Here's how the part is built. I have some questions about the finished solid (model axes, mm). Face numbers are marked on the shaded views. Give positions to 0.01 mm unless a question says otherwise; leave off trailing zeros. Order: outer loops, then holes, each group sorted by start corner. A loop starts at its lowest first (then second) coordinate and runs counter-clockwise, first axis right, second up. Notation, with made-up numbers: (-9.75, 89.5) -> (35.25, 89.5) arc R18 ccw to (35.25, 121.5) -> close; hole circle Ø8 at (-23, 51). An arc over 180 degrees is marked (long way). Write each question's results on one line, items separated by ' | '. Start each with the question number.
Q1. I'm going to push flat-ended pins straight in: pin 1 (1.4 mm diameter, centred on x = 10.2, y = 5.063, fed in from +Z); pin 2 (3.5 mm diameter, centred on x = 6, y = 9.5, fed in from +Z). Where does each tip first touch, or does it pass through?
Q2. Imagine slicing it at B-B, the plane y = 29.21. Please give me the cut outline in (x, z).
Q3. I need wall thicknesses on line 1 along Y through (x, z) = (17.5, -1.1); line 2 along X through (y, z) = (1, -1.25); line 3 along Y through (x, z) = (2, -3.05). Which ranges of each line are inside material? Lowest first, please. Write a range as [from, to].
Q4. Imagine slicing it at D-D, the plane y = 13. Please give me the cut outline in (x, z), then the cut area to 3 significant figures.
Q5. Imagine slicing it at C-C, the plane z = -3.2. Please give me the cut outline in (x, y).
Q6. Imagine slicing it at A-A, the plane x = 22.86. Please give me the cut outline in (y, z).
Q7. Thinking about a two-plate mould opening in Z: for the marked faces 1, 2 and 3, which applies, pulls with the +Z half, pulls with the -Z half, needs draft (parallel to the pull), parting line crosses it, or undercut?
```python
from build123d import *

# Parameters (mm, degrees)
PAD_DEPTH       = 3.2
THICKNESS001_T  = -2
SKETCH010_R     = 1.25
POCKET002_DEPTH = 2.001
SKETCH011_R     = 1.5
SKETCH011_R_2   = 1.2
POCKET003_DEPTH = 1


with BuildPart() as part:
    # Sketch009 → Pad (new body)
    with BuildSketch(Plane.XY):
        with BuildLine():
            Line((-2.4, 31.749999), (-2.4, 0))
            ThreePointArc((-2.4, 0), (-1.697056, -1.697056), (0, -2.4))
            Line((0, -2.4), (25.4, -2.4))
            ThreePointArc((25.4, -2.4), (27.097056, -1.697057), (27.8, -1e-06))
            Line((27.8, -1e-06), (27.8, 31.75))
            ThreePointArc((27.8, 31.75), (27.097057, 33.447056), (25.400001, 34.15))
            Line((25.400001, 34.15), (1e-06, 34.15))
            ThreePointArc((1e-06, 34.15), (-1.697056, 33.447056), (-2.4, 31.749999))
        make_face()
    extrude(amount=PAD_DEPTH)

    # Thickness001
    thickness001_openings = [part.faces().sort_by_distance(p)[0] for p in [
        (12.7, 15.875, 3.2),
    ]]
    offset(amount=THICKNESS001_T, openings=thickness001_openings)

    # Sketch010 (on Face19 of Thickness001) → Pocket002 (cut, through all)
    with BuildSketch(Plane.XY.offset(2)):
        with Locations((2.54, 29.21)):
            Circle(SKETCH010_R)
        with Locations((22.86, 29.21)):
            Circle(SKETCH010_R)
        with Locations((22.86, 2.54)):
            Circle(SKETCH010_R)
        with Locations((2.54, 2.54)):
            Circle(SKETCH010_R)
    extrude(amount=-POCKET002_DEPTH, mode=Mode.SUBTRACT)

    # Sketch011 (on Face23 of Pocket002) → Pocket003 (cut)
    with BuildSketch(Plane.XY.offset(2)):
        with Locations((9.45, 24.043)):
            Circle(SKETCH011_R)
        with Locations((15.95, 24.043)):
            Circle(SKETCH011_R)
        with Locations((15.95, 19.543)):
            Circle(SKETCH011_R)
        with Locations((19.025, 18.793)):
            Circle(SKETCH011_R)
        with Locations((19.025, 8.793)):
            Circle(SKETCH011_R)
        with Locations((9.45, 19.543)):
            Circle(SKETCH011_R)
        with Locations((6.375, 18.793)):
            Circle(SKETCH011_R)
        with Locations((6.375, 8.793)):
            Circle(SKETCH011_R)
        with Locations((3.97, 16.293)):
            Circle(SKETCH011_R_2)
        with Locations((3.97, 13.793)):
            Circle(SKETCH011_R_2)
        with Locations((3.97, 11.293)):
            Circle(SKETCH011_R_2)
        with Locations((10.2, 5.063)):
            Circle(SKETCH011_R_2)
        with Locations((12.7, 5.063)):
            Circle(SKETCH011_R_2)
        with Locations((15.2, 5.063)):
            Circle(SKETCH011_R_2)
    extrude(amount=-POCKET003_DEPTH, mode=Mode.SUBTRACT)


with BuildPart() as part_1:
    # Body placement: moved
    add(part.part.moved(Location((0, 0, -3.6))))


solid = part_1.part
```
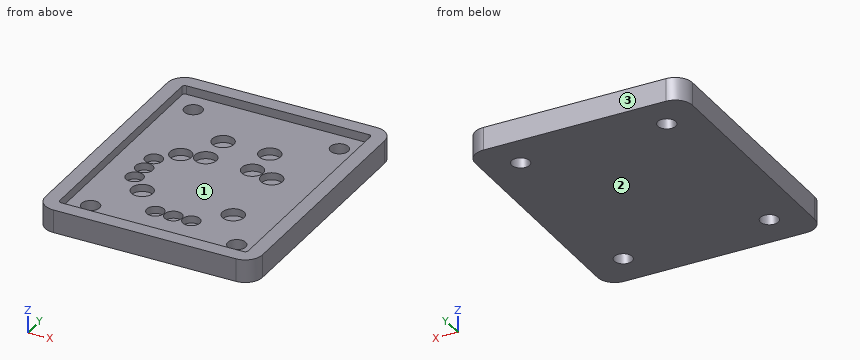
Geometry check:
1) pin 1: z = -2.6 | pin 2: z = -1.6
2) outline: (-2.4, -3.6) -> (1.29, -3.6) -> (1.29, -1.6) -> (-0.4, -1.6) -> (-0.4, -0.4) -> (-2.4, -0.4) -> close; (3.79, -3.6) -> (21.61, -3.6) -> (21.61, -1.6) -> (3.79, -1.6) -> close; (24.11, -3.6) -> (27.8, -3.6) -> (27.8, -0.4) -> (25.8, -0.4) -> (25.8, -1.6) -> (24.11, -1.6) -> close
3) line 1: [-2.4, -0.4], [32.15, 34.15] | line 2: [-2.4, -0.4], [25.8, 27.8] | line 3: [-2.4, 1.41], [3.67, 28.08], [30.34, 34.15]
4) outline: (-2.4, -3.6) -> (27.8, -3.6) -> (27.8, -0.4) -> (25.8, -0.4) -> (25.8, -1.6) -> (4.87, -1.6) -> (4.87, -2.6) -> (3.07, -2.6) -> (3.07, -1.6) -> (-0.4, -1.6) -> (-0.4, -0.4) -> (-2.4, -0.4) -> close | area: 63.4 mm²
5) outline: (-2.4, 0) arc R2.4 ccw to (0, -2.4) -> (25.4, -2.4) arc R2.4 ccw to (27.8, 0) -> (27.8, 31.75) arc R2.4 ccw to (25.4, 34.15) -> (0, 34.15) arc R2.4 ccw to (-2.4, 31.75) -> close; hole circle Ø2.5 at (2.54, 2.54); hole circle Ø2.5 at (2.54, 29.21); hole circle Ø2.5 at (22.86, 2.54); hole circle Ø2.5 at (22.86, 29.21)
6) outline: (-2.4, -3.6) -> (1.29, -3.6) -> (1.29, -1.6) -> (-0.4, -1.6) -> (-0.4, -0.4) -> (-2.4, -0.4) -> close; (3.79, -3.6) -> (27.96, -3.6) -> (27.96, -1.6) -> (3.79, -1.6) -> close; (30.46, -3.6) -> (34.15, -3.6) -> (34.15, -0.4) -> (32.15, -0.4) -> (32.15, -1.6) -> (30.46, -1.6) -> close
7) face 1: pulls with the +Z half | face 2: pulls with the -Z half | face 3: needs draft
